Geometry: final body of the model. Coordinates: model frame, mm. Face numbers are marked on the shaded views. Give positions to 0.01 mm unless a question says otherwise; leave off trailing zeros. Write each loop counter-clockwise with the first axis right and the second up, starting at its lowest first coordinate (ties: lowest second). Pieces come first, ordered by that corner, then holes. Notation, with made-up numbers: M 57.5,-37.5 L 92.5,-37.5 A35 ccw 92.5,-3.5 Z; hole C 7.25,-4.75 d9. An arc over 180 degrees is marked long. Answer as a JSON object with one key per item and string values.
from build123d import *

# Parameters (mm, degrees)
F0_R         = 10
F0_R_2       = 7.5
F1_DEPTH     = 10
F2_W         = 50
F2_H         = 42
F2_R         = 7.5
F3_DEPTH     = 5
F4_T1_DEPTH  = 123.8
F4_T3_DEPTH  = 11.5
F4_T5_DEPTH  = 23.6
F4_T7_DEPTH  = 22
F4_T9_DEPTH  = 11.5
F4_T11_DEPTH = 23.6
F4_T14_ANGLE = 71.0490813257
F4_T16_ANGLE = 71.0490813257
F4_T18_ANGLE = 71.0490813257
F4_T20_ANGLE = 71.0490813257
F4_T25_DEPTH = 19
F4_T29_DEPTH = 131.3
F4_T36_DEPTH = 131.3
F4_T40_DEPTH = 19
F4_T47_DEPTH = 19
F4_T51_DEPTH = 131.3
F4_T58_DEPTH = 131.3
F4_T62_DEPTH = 19


# Not quite as in the source:
# - a fillet or chamfer that OpenCascade refuses, or shapes differently, is made with other operations: its cross-section is extruded or revolved along the edge and cut away or added


with BuildPart() as f1:
    # F0 (on Front) → F1 (new body)
    with BuildSketch(Plane.XZ):
        with BuildLine():
            ThreePointArc((126, 3.5), (95.5089399385, 7.1742403064), (70.5, 25))
            Line((70.5, 25), (61.9, 25))
            Line((61.9, 25), (61.9, 21))
            Line((61.9, 21), (-61.9, 21))
            Line((-61.9, 21), (-61.9, 25))
            Line((-61.9, 25), (-70.5, 25))
            ThreePointArc((-70.5, 25), (-95.5089399385, 7.1742403064), (-126, 3.5))
            Line((-126, 3.5), (-126, -3.5))
            ThreePointArc((-126, -3.5), (-95.5089399385, -7.1742403064), (-70.5, -25))
            Line((-70.5, -25), (-61.9, -25))
            Line((-61.9, -25), (-61.9, -21))
            Line((-61.9, -21), (61.9, -21))
            Line((61.9, -21), (61.9, -25))
            Line((61.9, -25), (70.5, -25))
            ThreePointArc((70.5, -25), (95.5089399385, -7.1742403064), (126, -3.5))
            Line((126, -3.5), (126, 3.5))
        make_face()
        with Locations((-76, 0)):
            Circle(F0_R, mode=Mode.SUBTRACT)
        Circle(F0_R_2, mode=Mode.SUBTRACT)
        with Locations((76, 0)):
            Circle(F0_R, mode=Mode.SUBTRACT)
    extrude(amount=F1_DEPTH)

    # F2 (on face) → F3 (cut)
    with BuildSketch(Plane(origin=(0, 0, 0), x_dir=(-1, 0, 0), z_dir=(0, 1, 0))):
        Rectangle(F2_W, F2_H)
        Circle(F2_R, mode=Mode.SUBTRACT)
    extrude(amount=-F3_DEPTH, mode=Mode.SUBTRACT)

    # F4: fillet of radius 3 on 16 edges, made by hand

    # F4_s2 → F4_t1 (cut)
    with BuildSketch(Plane.YZ.offset(-61.9)):
        with BuildLine():
            ThreePointArc((-10, -18), (-9.1213203436, -20.1213203436), (-7, -21))
            Line((-7, -21), (-10, -21))
            Line((-10, -21), (-10, -18))
        make_face()
        with BuildLine():
            ThreePointArc((-10, 18), (-9.1213203436, 20.1213203436), (-7, 21))
            Line((-7, 21), (-10, 21))
            Line((-10, 21), (-10, 18))
        make_face()
    extrude(amount=F4_T1_DEPTH, mode=Mode.SUBTRACT)

    # F4_s4 → F4_t3 (cut)
    with BuildSketch(Plane.XY.offset(-32.5)):
        with BuildLine():
            ThreePointArc((64.9, -10), (62.7786796564, -9.1213203436), (61.9, -7))
            Line((61.9, -7), (61.9, -10))
            Line((61.9, -10), (64.9, -10))
        make_face()
        with BuildLine():
            ThreePointArc((-64.9, -10), (-62.7786796564, -9.1213203436), (-61.9, -7))
            Line((-61.9, -7), (-61.9, -10))
            Line((-61.9, -10), (-64.9, -10))
        make_face()
    extrude(amount=F4_T3_DEPTH, mode=Mode.SUBTRACT)

    # F4_s6 → F4_t5 (cut)
    with BuildSketch(Plane.YZ.offset(54.4)):
        with BuildLine():
            ThreePointArc((-10, -22), (-9.1213203436, -24.1213203436), (-7, -25))
            Line((-7, -25), (-10, -25))
            Line((-10, -25), (-10, -22))
        make_face()
        with BuildLine():
            ThreePointArc((-10, 22), (-9.1213203436, 24.1213203436), (-7, 25))
            Line((-7, 25), (-10, 25))
            Line((-10, 25), (-10, 22))
        make_face()
    extrude(amount=F4_T5_DEPTH, mode=Mode.SUBTRACT)

    # F4_s8 → F4_t7 (cut)
    with BuildSketch(Plane.XY.offset(-11)):
        with BuildLine():
            ThreePointArc((123, -10), (125.1213203436, -9.1213203436), (126, -7))
            Line((126, -7), (126, -10))
            Line((126, -10), (123, -10))
        make_face()
        with BuildLine():
            ThreePointArc((-123, 0), (-125.1213203436, -0.8786796564), (-126, -3))
            Line((-126, -3), (-126, 0))
            Line((-126, 0), (-123, 0))
        make_face()
    extrude(amount=F4_T7_DEPTH, mode=Mode.SUBTRACT)

    # F4_s10 → F4_t9 (cut)
    with BuildSketch(Plane.XY.offset(21)):
        with BuildLine():
            ThreePointArc((64.9, -10), (62.7786796564, -9.1213203436), (61.9, -7))
            Line((61.9, -7), (61.9, -10))
            Line((61.9, -10), (64.9, -10))
        make_face()
        with BuildLine():
            ThreePointArc((-64.9, -10), (-62.7786796564, -9.1213203436), (-61.9, -7))
            Line((-61.9, -7), (-61.9, -10))
            Line((-61.9, -10), (-64.9, -10))
        make_face()
    extrude(amount=F4_T9_DEPTH, mode=Mode.SUBTRACT)

    # F4_s12 → F4_t11 (cut)
    with BuildSketch(Plane.YZ.offset(-78)):
        with BuildLine():
            ThreePointArc((-10, 22), (-9.1213203436, 24.1213203436), (-7, 25))
            Line((-7, 25), (-10, 25))
            Line((-10, 25), (-10, 22))
        make_face()
        with BuildLine():
            ThreePointArc((-10, -22), (-9.1213203436, -24.1213203436), (-7, -25))
            Line((-7, -25), (-10, -25))
            Line((-10, -25), (-10, -22))
        make_face()
    extrude(amount=F4_T11_DEPTH, mode=Mode.SUBTRACT)

    # F4_s13 → F4_t14 (revolve, cut)
    with BuildSketch(Plane(origin=(5.6700188901, 0, 8.6318707647), x_dir=(0, 1, 0), z_dir=(-0.5490187323, 0, -0.8358100452))):
        with BuildLine():
            ThreePointArc((-10, 69.1979444633), (-9.1213203436, 71.3192648069), (-7, 72.1979444633))
            Line((-7, 72.1979444633), (-10, 72.1979444633))
            Line((-10, 72.1979444633), (-10, 69.1979444633))
        make_face()
    revolve(axis=Axis((117.9593619468, -10, -65.127655258), (0, 1, 0)), revolution_arc=F4_T14_ANGLE, mode=Mode.SUBTRACT)

    # F4_s15 → F4_t16 (revolve, cut)
    with BuildSketch(Plane(origin=(126.3513869763, 0, 32.3212006938), x_dir=(0, 1, 0), z_dir=(0.9688050004, 0, 0.2478242748))):
        with BuildLine():
            ThreePointArc((-7, -28.2871731549), (-9.1213203436, -29.1658528113), (-10, -31.2871731549))
            Line((-10, -31.2871731549), (-10, -28.2871731549))
            Line((-10, -28.2871731549), (-7, -28.2871731549))
        make_face()
    revolve(axis=Axis((117.9593619468, -10, 65.127655258), (0, 1, 0)), revolution_arc=F4_T16_ANGLE, mode=Mode.SUBTRACT)

    # F4_s17 → F4_t18 (revolve, cut)
    with BuildSketch(Plane(origin=(-5.6700188901, 0, -8.6318707647), x_dir=(0, 1, 0), z_dir=(0.5490187323, 0, 0.8358100452))):
        with BuildLine():
            ThreePointArc((-10, 69.1979444633), (-9.1213203436, 71.3192648069), (-7, 72.1979444633))
            Line((-7, 72.1979444633), (-10, 72.1979444633))
            Line((-10, 72.1979444633), (-10, 69.1979444633))
        make_face()
    revolve(axis=Axis((-117.9593619468, -10, 65.127655258), (0, 1, 0)), revolution_arc=F4_T18_ANGLE, mode=Mode.SUBTRACT)

    # F4_s19 → F4_t20 (revolve, cut)
    with BuildSketch(Plane(origin=(-126.3513869763, 0, -32.3212006938), x_dir=(0, 1, 0), z_dir=(-0.9688050004, 0, -0.2478242748))):
        with BuildLine():
            ThreePointArc((-10, -31.2871731549), (-9.1213203436, -29.1658528113), (-7, -28.2871731549))
            Line((-7, -28.2871731549), (-10, -28.2871731549))
            Line((-10, -28.2871731549), (-10, -31.2871731549))
        make_face()
    revolve(axis=Axis((-117.9593619468, -10, -65.127655258), (0, 1, 0)), revolution_arc=F4_T20_ANGLE, mode=Mode.SUBTRACT)


with BuildPart() as f4_tool23:
    # F4_s24 → F4_t25 (new body)
    with BuildSketch(Plane.XY.offset(-32.5)):
        with BuildLine():
            ThreePointArc((-64.9, -10), (-62.7786796564, -9.1213203436), (-61.9, -7))
            Line((-61.9, -7), (-61.9, -10))
            Line((-61.9, -10), (-64.9, -10))
        make_face()
    extrude(amount=F4_T25_DEPTH)

    split(bisect_by=Plane.XY.offset(-21), keep=Keep.TOP)


with BuildPart() as f4_tool27:
    # F4_s28 → F4_t29 (new body)
    with BuildSketch(Plane.YZ.offset(-69.4)):
        with BuildLine():
            ThreePointArc((-10, -18), (-9.1213203436, -20.1213203436), (-7, -21))
            Line((-7, -21), (-10, -21))
            Line((-10, -21), (-10, -18))
        make_face()
    extrude(amount=F4_T29_DEPTH)

    split(bisect_by=Plane.YZ.offset(-61.9), keep=Keep.BOTTOM)


with BuildPart() as f4_tool23_1:
    add(f4_tool23.part)

    # F4_t31: intersect F4_tool27
    add(f4_tool27.part, mode=Mode.INTERSECT)


with BuildPart() as f1_1:
    add(f1.part)

    # F4_t21: cut F4_tool23
    add(f4_tool23_1.part, mode=Mode.SUBTRACT)


with BuildPart() as f4_tool34:
    # F4_s35 → F4_t36 (new body)
    with BuildSketch(Plane.YZ.offset(-61.9)):
        with BuildLine():
            ThreePointArc((-10, -18), (-9.1213203436, -20.1213203436), (-7, -21))
            Line((-7, -21), (-10, -21))
            Line((-10, -21), (-10, -18))
        make_face()
    extrude(amount=F4_T36_DEPTH)

    split(bisect_by=Plane.YZ.offset(61.9), keep=Keep.TOP)


with BuildPart() as f4_tool38:
    # F4_s39 → F4_t40 (new body)
    with BuildSketch(Plane.XY.offset(-13.5)):
        with BuildLine():
            ThreePointArc((64.9, -10), (62.7786796564, -9.1213203436), (61.9, -7))
            Line((61.9, -7), (61.9, -10))
            Line((61.9, -10), (64.9, -10))
        make_face()
    extrude(amount=-F4_T40_DEPTH)

    split(bisect_by=Plane.XY.offset(-21), keep=Keep.TOP)


with BuildPart() as f4_tool34_1:
    add(f4_tool34.part)

    # F4_t42: intersect F4_tool38
    add(f4_tool38.part, mode=Mode.INTERSECT)


with BuildPart() as f1_2:
    add(f1_1.part)

    # F4_t32: cut F4_tool34
    add(f4_tool34_1.part, mode=Mode.SUBTRACT)


with BuildPart() as f4_tool45:
    # F4_s46 → F4_t47 (new body)
    with BuildSketch(Plane.XY.offset(32.5)):
        with BuildLine():
            ThreePointArc((64.9, -10), (62.7786796564, -9.1213203436), (61.9, -7))
            Line((61.9, -7), (61.9, -10))
            Line((61.9, -10), (64.9, -10))
        make_face()
    extrude(amount=-F4_T47_DEPTH)

    split(bisect_by=Plane.XY.offset(21), keep=Keep.BOTTOM)


with BuildPart() as f4_tool49:
    # F4_s50 → F4_t51 (new body)
    with BuildSketch(Plane.YZ.offset(69.4)):
        with BuildLine():
            ThreePointArc((-10, 18), (-9.1213203436, 20.1213203436), (-7, 21))
            Line((-7, 21), (-10, 21))
            Line((-10, 21), (-10, 18))
        make_face()
    extrude(amount=-F4_T51_DEPTH)

    split(bisect_by=Plane.YZ.offset(61.9), keep=Keep.TOP)


with BuildPart() as f4_tool45_1:
    add(f4_tool45.part)

    # F4_t53: intersect F4_tool49
    add(f4_tool49.part, mode=Mode.INTERSECT)


with BuildPart() as f1_3:
    add(f1_2.part)

    # F4_t43: cut F4_tool45
    add(f4_tool45_1.part, mode=Mode.SUBTRACT)


with BuildPart() as f4_tool56:
    # F4_s57 → F4_t58 (new body)
    with BuildSketch(Plane.YZ.offset(61.9)):
        with BuildLine():
            ThreePointArc((-10, 18), (-9.1213203436, 20.1213203436), (-7, 21))
            Line((-7, 21), (-10, 21))
            Line((-10, 21), (-10, 18))
        make_face()
    extrude(amount=-F4_T58_DEPTH)

    split(bisect_by=Plane.YZ.offset(-61.9), keep=Keep.BOTTOM)


with BuildPart() as f4_tool60:
    # F4_s61 → F4_t62 (new body)
    with BuildSketch(Plane.XY.offset(13.5)):
        with BuildLine():
            ThreePointArc((-64.9, -10), (-62.7786796564, -9.1213203436), (-61.9, -7))
            Line((-61.9, -7), (-61.9, -10))
            Line((-61.9, -10), (-64.9, -10))
        make_face()
    extrude(amount=F4_T62_DEPTH)

    split(bisect_by=Plane.XY.offset(21), keep=Keep.BOTTOM)


with BuildPart() as f4_tool56_1:
    add(f4_tool56.part)

    # F4_t64: intersect F4_tool60
    add(f4_tool60.part, mode=Mode.INTERSECT)


with BuildPart() as f1_4:
    add(f1_3.part)

    # F4_t54: cut F4_tool56
    add(f4_tool56_1.part, mode=Mode.SUBTRACT)


solid = f1_4.part
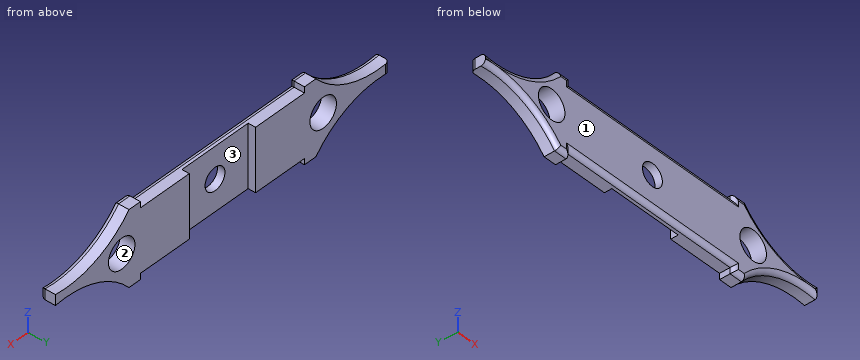
1) Cut plane A-A on x = 0. Return loops of the section in (y, z), and give its area (3 significant figures).
Geometry check:
{"outline": "M -10,-18 A3 ccw -7,-21 L -5,-21 L -5,-7.5 L -10,-7.5 Z; M -10,7.5 L -5,7.5 L -5,21 L -7,21 A3 ccw -10,18 Z", "area": "131 mm2"}
2) Pull-direction query (X, two-part tool) for the marked faces 1, 2 and 3; classes: pulls with the +X half, pulls with the -X half, needs draft (parallel to the pull), parting line crosses it, or undercut.
Geometry check:
{"face 1": "needs draft", "face 2": "undercut", "face 3": "undercut"}
3) Line query: line 1 (X direction, y = -1.5, z = 1.5); line 2 (X direction, y = -6.5, z = 1.5); line 3 (Z direction, x = -57.5, y = -1). Output: solid intervals per line, ascending. Write a range as from..to.
Geometry check:
{"line 1": "x = -125.6..-85.89, -66.11..-25, 25..66.11, 85.89..126", "line 2": "x = -126..-85.89, -66.11..-7.35, 7.35..66.11, 85.89..126", "line 3": "z = -21..21"}
4) Contact query for flat-ended pins moving along their axis: P1, Ø4.5, axis at y = -3, z = 22.5, coming from the +X side; P2, Ø5, axis at y = -5, z = -19.5, coming from the +X side; P3, Ø1, axis at y = -2, z = 19, coming from the -X side; P4, Ø9, axis at x = 0, z = 0, coming from the +Y side. Output: stop coordinate, or through.
Geometry check:
{"P1": "stops at x = 74.96", "P2": "stops at x = 78.64", "P3": "stops at x = -76.87", "P4": "passes through"}
5) Cut plane B-B on x = 40.5. Return loops of the section in (y, z), and give its area (3 significant figures).
Geometry check:
{"outline": "M -10,-18 A3 ccw -7,-21 L 0,-21 L 0,21 L -7,21 A3 ccw -10,18 Z", "area": "416 mm2"}
